Verification items for this drawing (mm, ordinates from the low corner). A direction names the side the tool comes from. Give positions to 0.01 mm unless a question says otherwise; leave off trailing zeros. Loops run counter-clockwise (first coordinate to the right, second up) from the corner with the lowest first, then second, coordinate; pieces in that order, holes last. Notation, with made-up numbers: (28, 81) -> (45, 81) arc R27 ccw to (45, 103) -> close; hole circle Ø9 at (-22, -12.5). An arc over 180 degrees is marked (long way). Answer in a Markdown table with one row per item. Add a question column.
Q1. Material ranges on probe 1 along X at (y, z) = (6.5, 8.75); probe 2 along X at (y, z) = (4, 4); probe 3 along Y at (x, z) = (8.25, 2.75) (1 decimal), recorded low to high.
Q2. Section check D-D on x = 6. Give the number of separate pieces and of enclosed holes in the cut face, and give its area (3 significant figures).
Q3. Section check A-A on z = 7.5. Enter the section's corners in (x, y).
Q4. Release check for a two-part mould opening along Z. For the marked faces 1, 2 and 3 record: pulls with the +Z half, pulls with the -Z half, needs draft (parallel to the pull), parting line crosses it, or undercut.
Q5. Set-up check for the marked faces 4, 5 and 6: record each of +Z, -Z, +X, -X, +Y, -Y from which the full face is reachable in a straight line by a thin tool's end or side.
Q6. Gauge pin test, flat ends, axial feed: P1, Ø2, axis at y = 16, z = 7.5, coming from the +X side; P2, Ø3.5, axis at y = 16.5, z = 9, coming from the +X side. Record the tip position at first contact, or that the pin passes through.
Q7. Section check C-C on z = 1.5. Enter the section's corners in (x, y), and give its area (3 significant figures).
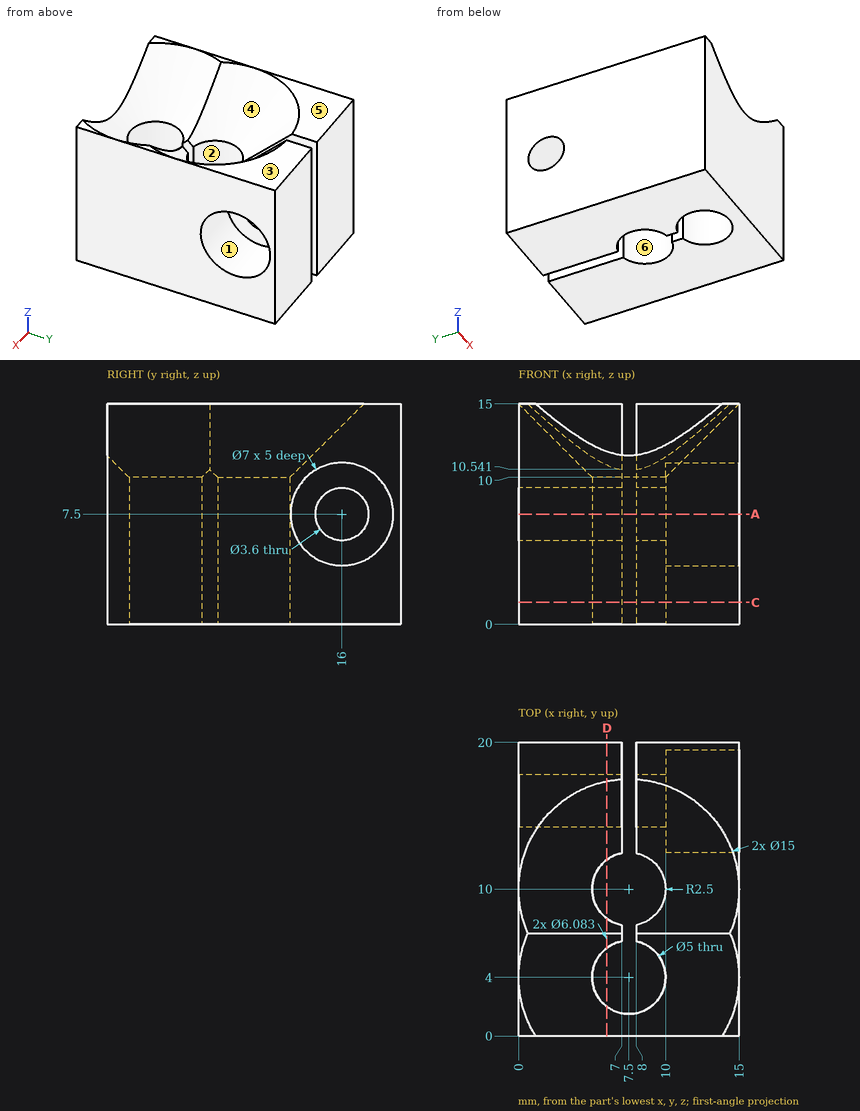
Taken from the geometry:
| question | item | result |
|---|---|---|
| 1 | probe 1 | x = 0 to 7, 8 to 15 |
| 1 | probe 2 | x = 0 to 5, 10 to 15 |
| 1 | probe 3 | y = 0 to 1.6, 6.4 to 7.6, 12.4 to 20 |
| 2 | separate pieces | 3 |
| 2 | enclosed holes | 1 |
| 2 | area | 139 mm² |
| 3 | outline | (0, 0) -> (15, 0) -> (15, 12.5) -> (10, 12.5) -> (10, 14.2) -> (8, 14.2) -> (8, 12.45) arc R2.5 cw to (8, 7.55) -> (8, 6.45) arc R2.5 cw (long way) to (7, 6.45) -> (7, 7.55) arc R2.5 cw to (7, 12.45) -> (7, 14.2) -> (0, 14.2) -> close; (0, 17.8) -> (7, 17.8) -> (7, 20) -> (0, 20) -> close; (8, 17.8) -> (10, 17.8) -> (10, 19.5) -> (15, 19.5) -> (15, 20) -> (8, 20) -> close |
| 4 | face 1 | undercut |
| 4 | face 2 | needs draft |
| 4 | face 3 | pulls with the +Z half |
| 5 | face 4 | +Z |
| 5 | face 5 | +Z, +X, -X, +Y, -Y |
| 5 | face 6 | +Z, -Z |
| 6 | P1 | passes through |
| 6 | P2 | stops at x = 10 |
| 7 | outline | (0, 0) -> (15, 0) -> (15, 20) -> (8, 20) -> (8, 12.45) arc R2.5 cw to (8, 7.55) -> (8, 6.45) arc R2.5 cw (long way) to (7, 6.45) -> (7, 7.55) arc R2.5 cw to (7, 12.45) -> (7, 20) -> (0, 20) -> close |
| 7 | area | 252 mm² |
